Build history of the part. All positions in model axes, mm. A direction names the side the tool comes from. Coordinates: 2 decimals unless noted, no trailing zeros. Write each loop counter-clockwise with the first axis right and the second up, starting at its lowest first coordinate (ties: lowest second). Pieces come first, ordered by that corner, then holes. Notation, with made-up numbers: M 1,80.25 L 7,80.25 A22 ccw 7,98.25 Z; hole C -26.75,64.5 d5. An arc over 180 degrees is marked long. Use CSV: the item, a comma, the result in double quotes. Start each with the question number.
```python
from build123d import *

# Parameters (mm, degrees)
BOSS_EXTRUDE3_DEPTH = 3.81
SKETCH1_7_R         = 2.54
CUT_EXTRUDE6_DEPTH  = 3.81
CUT_EXTRUDE7_DEPTH  = 4.81
FILLET1_R           = 2.54
FILLET2_R           = 2.54


with BuildPart() as part:
    # Sketch1 → Boss-Extrude3 (new body)
    with BuildSketch(Plane.XY):
        Polygon((-103.210268441, 60.572134971), (-88.641426958, 81.378596896), (-25.4, 139.7), (0, 139.7), (88.9, 25.4), (88.9, 0), (-16.704294619, 0), align=None)
    extrude(amount=BOSS_EXTRUDE3_DEPTH)

    # Sketch1_7 → Cut-Extrude6 (cut)
    with BuildSketch(Plane.XY):
        with Locations((-12.7, 57.15)):
            Circle(SKETCH1_7_R)
        with Locations((-12.7, 69.85)):
            Circle(SKETCH1_7_R)
        with Locations((-12.7, 82.55)):
            Circle(SKETCH1_7_R)
        with Locations((-12.7, 95.25)):
            Circle(SKETCH1_7_R)
        with Locations((-12.7, 107.95)):
            Circle(SKETCH1_7_R)
        with Locations((-12.7, 120.65)):
            Circle(SKETCH1_7_R)
        with Locations((-12.7, 133.35)):
            Circle(SKETCH1_7_R)
        with Locations((6.35, 12.7)):
            Circle(SKETCH1_7_R)
        with Locations((19.05, 12.7)):
            Circle(SKETCH1_7_R)
        with Locations((31.75, 12.7)):
            Circle(SKETCH1_7_R)
        with Locations((44.45, 12.7)):
            Circle(SKETCH1_7_R)
        with Locations((57.15, 12.7)):
            Circle(SKETCH1_7_R)
        with Locations((69.85, 12.7)):
            Circle(SKETCH1_7_R)
        with Locations((82.55, 12.7)):
            Circle(SKETCH1_7_R)
        with Locations((-28.304846444, 23.626631112)):
            Circle(SKETCH1_7_R)
        with Locations((-38.708077406, 30.911051854)):
            Circle(SKETCH1_7_R)
        with Locations((-49.111308369, 38.195472596)):
            Circle(SKETCH1_7_R)
        with Locations((-59.514539331, 45.479893337)):
            Circle(SKETCH1_7_R)
        with Locations((-69.917770294, 52.764314079)):
            Circle(SKETCH1_7_R)
        with Locations((-80.321001256, 60.048734821)):
            Circle(SKETCH1_7_R)
        with Locations((-90.724232219, 67.333155562)):
            Circle(SKETCH1_7_R)
    extrude(amount=CUT_EXTRUDE6_DEPTH, mode=Mode.SUBTRACT)

    # Sketch2 → Cut-Extrude7 (cut, through all)
    with BuildSketch(Plane.XY.offset(3.81)):
        Polygon((-58.849974987, 101.941947594), (-37.140287646, 51.518645834), (-80.559662327, 81.92121929), align=None)
        Polygon((-30.48, 61.7413962), (-50.932108739, 109.243823775), (-30.48, 128.104809927), align=None)
        Polygon((5.094015595, 124.876135436), (5.178673612, 35.321443219), (38.137547923, 82.391593871), align=None)
        Polygon((10.283477792, 25.107422311), (44.656622028, 74.009927164), (79.029766265, 29.815884574), align=None)
    extrude(amount=-CUT_EXTRUDE7_DEPTH, mode=Mode.SUBTRACT)

    # Fillet1
    fillet1_edges = [part.edges().sort_by_distance(p)[0] for p in [
        (-30.48, 61.7413962, 1.905),
        (-50.932108739, 109.243823775, 1.905),
        (-30.48, 128.104809927, 1.905),
        (5.178673612, 35.321443219, 1.905),
        (5.094015595, 124.876135436, 1.905),
        (38.137547923, 82.391593871, 1.905),
        (10.283477792, 25.107422311, 1.905),
        (44.656622028, 74.009927164, 1.905),
        (79.029766265, 29.815884574, 1.905),
        (-58.849974987, 101.941947594, 1.905),
        (-37.140287646, 51.518645834, 1.905),
        (-80.559662327, 81.92121929, 1.905),
    ]]
    fillet(fillet1_edges, radius=FILLET1_R)

    # Fillet2
    fillet2_edges = [part.edges().sort_by_distance(p)[0] for p in [
        (0, 139.7, 1.905),
        (-25.4, 139.7, 1.905),
        (-88.641426958, 81.378596896, 1.905),
        (-103.210268441, 60.572134971, 1.905),
        (-16.704294619, 0, 1.905),
        (88.9, 0, 1.905),
        (88.9, 25.4, 1.905),
    ]]
    fillet(fillet2_edges, radius=FILLET2_R)


solid = part.part
```
1. Slice it at A-A (y = 12.7). Count the separate pieces of the cut face and the enclosed holes in it, and give its area (3 significant figures).
2. Slice it at B-B (x = 82.55). List the corners of the cut face in (y, z), and give its area (3 significant figures).
3. Pull direction X, two halves, no side cores. Call faces 3 (the flat face through (88.9, 14, 2)), 4 (the flat face through (-5, 55, 3.81)), 5 (the flat face through (-69.98, 91.68, 1.93)): pulls with the +X half, pulls with the -X half, needs draft (parallel to the pull), parting line crosses it, or undercut.
4. 3-axis set-ups, long thin cutter, end or side, ignore diameter. For faces 1 (the cylindrical face through (-59.269, 100.135, 1.878)), 2 (the flat face through (-95.37, 71.77, 1.88)): which of +Z, -Z, +X, -X, +Y, -Y reach the whole face in a straight line?
5. Drill centre lines: line 1 along X through (y, z) = (51, 3.4) (3 decimals); line 2 along X through (y, z) = (67, 3.2); line 3 along Y through (x, z) = (57, 3.2). Where is each one in solid material? Low to high. Write a range as from..to.
6. Slice it at C-C (x = 24). List the corners of the cut face in (y, z), and give its area (3 significant figures).
7. Flat gauge pins, fed straight in: pin 1 (1 mm diameter, centred on y = 25.5, z = 0.5, fed in from +X); pin 2 (1.5 mm diameter, centred on x = -76, z = 2, fed in from -Y). Where does each tip first touch, or does it go through?
Established:
1,separate pieces,"8"
1,enclosed holes,"0"
1,area,"336 mm2"
2,outline,"M 0,0 L 10.16,0 L 10.16,3.81 L 0,3.81 Z; M 15.24,0 L 33.56,0 L 33.56,3.81 L 15.24,3.81 Z"
2,area,"109 mm2"
3,face 3,"pulls with the +X half"
3,face 4,"needs draft"
3,face 5,"undercut"
4,face 1,"+Z, -Z"
4,face 2,"+Z, -Z, -X, +Y"
5,line 1,"x = -89.54..-71.745, -68.091..5.164, 16.157..28.483, 62.553..68.989"
5,line 2,"x = -98.71..-93.24, -88.21..-59.25, -43.81..5.15, 27.36..39.73, 50.11..56.54"
5,line 3,"y = 0..10.16, 15.24..28.31, 58.14..66.41"
6,outline,"M 0,0 L 26.05,0 L 26.05,3.81 L 0,3.81 Z; M 44.62,0 L 62.2,0 L 62.2,3.81 L 44.62,3.81 Z; M 100.57,0 L 108.84,0 L 108.84,3.81 L 100.57,3.81 Z"
6,area,"198 mm2"
7,pin 1,"stops at x = 88.86"
7,pin 2,"stops at y = 40.99"
